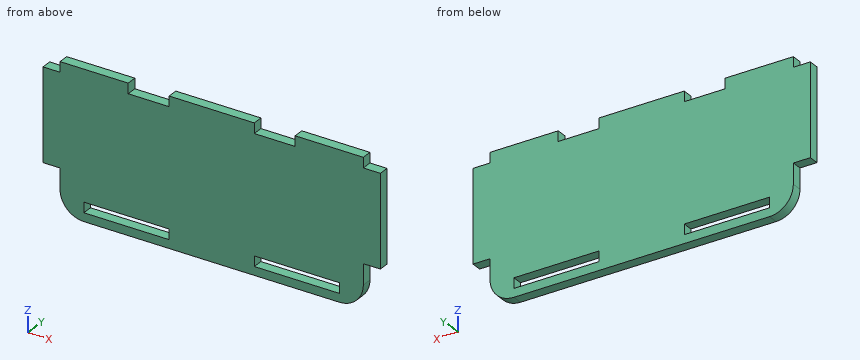
```python
from build123d import *

# Parameters (mm, degrees)
ESTRUSIONE_ESTRUSIONE1_DEPTH      = 30
ESTRUSIONE_ESTRUSIONE1_DEPTH_BACK = 3
SCHIZZO1_W                        = 89
SCHIZZO1_H                        = 3
SCHIZZO2_W                        = 12
SCHIZZO2_H                        = 3
TAGLIO_ESTRUSIONE1_DEPTH          = 10
SCHIZZO3_W                        = 27
SCHIZZO3_H                        = 3
ESTRUSIONE_ESTRUSIONE2_DEPTH      = 5
SCHIZZO4_W                        = 89
SCHIZZO4_H                        = 3
ESTRUSIONE_ESTRUSIONE3_DEPTH      = 10
SCHIZZO5_W                        = 25
SCHIZZO5_H                        = 3
TAGLIO_ESTRUSIONE2_DEPTH          = 8
RACCORDO1_R                       = 7


with BuildPart() as part:
    # Schizzo1 → Estrusione-Estrusione1 (new, two sides: drawn at the far end of the back side and taken through both)
    with BuildSketch(Plane.XY.offset(-ESTRUSIONE_ESTRUSIONE1_DEPTH_BACK)):
        with Locations((0, -22.5)):
            Rectangle(SCHIZZO1_W, SCHIZZO1_H)
    extrude(amount=ESTRUSIONE_ESTRUSIONE1_DEPTH + ESTRUSIONE_ESTRUSIONE1_DEPTH_BACK)

    # Schizzo2 → Taglio-Estrusione1 (cut)
    with BuildSketch(Plane(origin=(0, -21, 0), x_dir=(1, 0, 0), z_dir=(0, 1, 0))):
        with Locations((18.5, -28.5)):
            Rectangle(SCHIZZO2_W, SCHIZZO2_H)
        with Locations((-18.5, -28.5)):
            Rectangle(SCHIZZO2_W, SCHIZZO2_H)
    extrude(amount=-TAGLIO_ESTRUSIONE1_DEPTH, mode=Mode.SUBTRACT)

    # Schizzo3 → Estrusione-Estrusione2 (add)
    with BuildSketch(Plane(origin=(44.5, 0, 0), x_dir=(0, 0, -1), z_dir=(1, 0, 0))):
        with Locations((-13.5, -22.5)):
            Rectangle(SCHIZZO3_W, SCHIZZO3_H)
    estrusione_estrusione2 = extrude(amount=ESTRUSIONE_ESTRUSIONE2_DEPTH)

    # Specchia1: Estrusione-Estrusione2 across plane
    add(estrusione_estrusione2.mirror(Plane(origin=(0, 0, 0), x_dir=(0, 0, 1), z_dir=(1, 0, 0))))

    # Schizzo4 → Estrusione-Estrusione3 (add)
    with BuildSketch(Plane(origin=(0, 0, -3), x_dir=(-1, 0, 0), z_dir=(0, 0, -1))):
        with Locations((0, -22.5)):
            Rectangle(SCHIZZO4_W, SCHIZZO4_H)
    extrude(amount=ESTRUSIONE_ESTRUSIONE3_DEPTH)

    # Schizzo5 → Taglio-Estrusione2 (cut)
    with BuildSketch(Plane(origin=(0, -21, 0), x_dir=(1, 0, 0), z_dir=(0, 1, 0))):
        with Locations((-25, 9)):
            Rectangle(SCHIZZO5_W, SCHIZZO5_H)
        with Locations((25, 9)):
            Rectangle(SCHIZZO5_W, SCHIZZO5_H)
    extrude(amount=-TAGLIO_ESTRUSIONE2_DEPTH, mode=Mode.SUBTRACT)

    # Raccordo1
    raccordo1_edges = [part.edges().sort_by_distance(p)[0] for p in [
        (-44.5, -22.5, -13),
        (44.5, -22.5, -13),
    ]]
    fillet(raccordo1_edges, radius=RACCORDO1_R)


solid = part.part
```
CAD build for the part. Positions are in the model's coordinates, mm. Round coordinates to 2 decimals unless told otherwise and drop trailing zeros. Write each loop counter-clockwise with the first axis right and the second up, starting at its lowest first coordinate (ties: lowest second). Pieces come first, ordered by that corner, then holes.
Item 1: Drill centre lines: L1, parallel to Z at x = 20, y = -23.2; L2, parallel to Z at x = 25.5, y = -21.35; L3, parallel to X at y = -23.1, z = -5. Where is each one in solid material? Low to high.
Filled in:
L1: z = -13 to -10.5, -7.5 to 27
L2: z = -13 to -10.5, -7.5 to 30
L3: x = -44.5 to 44.5
Item 2: Band-saw the part on D-D on z = -3. Write the cut outline in (x, y), then the cut area to 3 significant figures.
Filled in:
outline: (-44.5, -24) - (44.5, -24) - (44.5, -21) - (-44.5, -21) - close
area: 267 mm2
Item 3: Band-saw the part on B-B on y = -23.5. Give the number of separate pieces and of enclosed holes in the cut face, then the cut area to 3 significant figures.
Filled in:
separate pieces: 1
enclosed holes: 2
area: 3,850 mm2
Item 4: Band-saw the part on C-C on z = -9. Write the cut outline in (x, y), then the cut area to 3 significant figures.
Filled in:
outline: (-43.82, -24) - (-37.5, -24) - (-37.5, -21) - (-43.82, -21) - close; (-12.5, -24) - (12.5, -24) - (12.5, -21) - (-12.5, -21) - close; (37.5, -24) - (43.82, -24) - (43.82, -21) - (37.5, -21) - close
area: 113 mm2
Item 5: Drop flat-ended pins along their axis: pin 1 Ø0.9 at (y, z) = (-23, 28.5) entering from -X; pin 2 Ø1.5 at (x, y) = (-47, -22.5) entering from -Z; pin 3 Ø0.9 at (y, z) = (-22, -8.5) entering from -X. Give the stop position or say it passes through.
Filled in:
pin 1: stops at x = -44.5
pin 2: stops at z = 0
pin 3: stops at x = -44.19
Item 6: Band-saw the part on A-A on x = -15.5. Write the cut outline in (y, z), then the cut area to 3 significant figures.
Filled in:
outline: (-24, -13) - (-21, -13) - (-21, -10.5) - (-24, -10.5) - close; (-24, -7.5) - (-21, -7.5) - (-21, 27) - (-24, 27) - close
area: 111 mm2
